The model under review builds one solid part; all positions refer to its coordinate system, in mm. Coordinates: 2 decimals unless noted, no trailing zeros. Write item = value, one per line. Start each with the question number.
Q1. Clearance check with flat-ended pins moving along their axes: pin 1 Ø13 at (x, z) = (32, 718.5) entering from +Y; pin 2 Ø6 at (x, y) = (48, 19) entering from -Z; pin 3 Ø6 at (x, z) = (32, 681.5) entering from -Y. State where each tip first meets the part, or that it passes through.
Q2. Wall thickness on probe 1 along Z at (x, y) = (15.5, 26); probe 2 along Z at (x, y) = (28, 22.5); probe 3 along Z at (x, y) = (30, 8): over which ranges is each line inside the solid? List them lowest first.
Q3. Mouldability with a two-part tool opening along Z and no side actions: class faces 1 (the face through (31, 19, 1400)), 2 (the face through (31, 19, 0)), 3 (the face through (31, 23, 699)), 4 (the face through (31, 38, 1064)) as released by +Z, released by -Z, zero draft, split by the parting line, or undercut.
from build123d import *

# Parameters (mm, degrees)
ESQUISSE1_W             = 63
ESQUISSE1_H             = 38
BOSS_EXTRU_1_DEPTH      = 1400
ESQUISSE2_R             = 5
ENL_V_MAT_EXTRU_1_DEPTH = 50
ENL_V_START             = -1350
ESQUISSE2_2_R           = 5
ENL_V_MAT_EXTRU_2_DEPTH = 50
ESQUISSE3_W             = 63
ESQUISSE3_H             = 75
ENL_V_MAT_EXTRU_3_DEPTH = 15
ESQUISSE4_R             = 5
ENL_V_MAT_EXTRU_4_DEPTH = 1402.60550798


with BuildPart() as part:
    # Esquisse1 → Boss.-Extru.1 (new body)
    with BuildSketch(Plane.XY):
        with Locations((31.5, 19)):
            Rectangle(ESQUISSE1_W, ESQUISSE1_H)
    extrude(amount=BOSS_EXTRU_1_DEPTH)

    # Esquisse2 → Enlèv. mat.-Extru.1 (cut)
    with BuildSketch(Plane.XY.offset(1400)):
        with Locations((15, 19)):
            Circle(ESQUISSE2_R)
        with Locations(Location((48, 19, 0), (0, 0, 180))):
            Circle(ESQUISSE2_R)
    extrude(amount=-ENL_V_MAT_EXTRU_1_DEPTH, mode=Mode.SUBTRACT)

    # Esquisse2<2> → Enlèv. mat.-Extru.2 (cut)
    with BuildSketch(Plane.XY.offset(1400).offset(ENL_V_START)):
        with Locations((15, 19)):
            Circle(ESQUISSE2_2_R)
        with Locations(Location((48, 19, 0), (0, 0, 180))):
            Circle(ESQUISSE2_2_R)
    extrude(amount=-ENL_V_MAT_EXTRU_2_DEPTH, mode=Mode.SUBTRACT)

    # Esquisse3 → Enlèv. mat.-Extru.3 (cut)
    with BuildSketch(Plane(origin=(0, 38, 0), x_dir=(1, 0, 0), z_dir=(0, 1, 0))):
        with Locations((31.5, -700)):
            Rectangle(ESQUISSE3_W, ESQUISSE3_H)
    extrude(amount=-ENL_V_MAT_EXTRU_3_DEPTH, mode=Mode.SUBTRACT)

    # Esquisse4 → Enlèv. mat.-Extru.4 (cut, through all)
    with BuildSketch(Plane(origin=(0, 23, 0), x_dir=(1, 0, 0), z_dir=(0, 1, 0))):
        with Locations(Location((32, -718.5, 0), (0, 0, 270))):
            Circle(ESQUISSE4_R)
        with Locations(Location((32, -681.5, 0), (0, 0, 90))):
            Circle(ESQUISSE4_R)
    extrude(amount=-ENL_V_MAT_EXTRU_4_DEPTH, mode=Mode.SUBTRACT)


solid = part.part
Returned:
q1.pin_1 = 23
q1.pin_2 = 50
q1.pin_3 = through
q2.probe_1 = 0 to 662.5, 737.5 to 1400
q2.probe_2 = 0 to 678.5, 684.5 to 715.5, 721.5 to 1400
q2.probe_3 = 0 to 676.92, 686.08 to 713.92, 723.08 to 1400
q3.face_1 = released by +Z
q3.face_2 = released by -Z
q3.face_3 = undercut
q3.face_4 = zero draft
